from build123d import *

# Parameters (mm, degrees)
F0_W           = 80
F0_H           = 80
F1_DEPTH       = 80
F3_DEPTH       = 86.9
F4_W           = 8
F4_H           = 80
F5_DEPTH       = 25
F6_W           = 30
F6_H           = 25
F7_DEPTH       = 25
F9_DEPTH       = 50.3
F11_W          = 223.7579002976
F11_H          = 231.868326664
F12_DEPTH      = 25
F13_W          = 207.2095647454
F13_H          = 262.1310725808
F14_DEPTH      = 25
F16_DEPTH      = 127.5
F18_DEPTH      = 40.001
F18_DEPTH_BACK = 40.001


# Not quite as in the source:
# - a feature of the source that left no trace in its solid (it failed there, or was rolled back) is left out


with BuildPart() as f1:
    # F0 (on Top) → F1 (new body)
    with BuildSketch(Plane.XY):
        Rectangle(F0_W, F0_H)
    extrude(amount=F1_DEPTH)

    # F2 (on face) → F3 (cut)
    with BuildSketch(Plane.XZ.offset(40)):
        Polygon((-40, 28.6014117301), (0, 80), (-40, 80), align=None)
    extrude(amount=-F3_DEPTH, mode=Mode.SUBTRACT)

    # F4 (on face) → F5 (cut)
    with BuildSketch(Plane.XY.offset(80)):
        with Locations((9.4103766605, 0)):
            Rectangle(F4_W, F4_H)
    extrude(amount=-F5_DEPTH, mode=Mode.SUBTRACT)

    # F6 (on face) → F7 (cut)
    with BuildSketch(Plane.YZ.offset(5.4103766605)):
        with Locations((-25, 67.5)):
            Rectangle(F6_W, F6_H)
        with Locations((25, 67.5)):
            Rectangle(F6_W, F6_H)
    extrude(amount=-F7_DEPTH, mode=Mode.SUBTRACT)

    # F8 (on face) → F9 (cut)
    with BuildSketch(Plane(origin=(-40, 0, 0), x_dir=(0, -1, 0), z_dir=(-1, 0, 0))):
        Polygon((-10.1708276197, 55.0271123648), (0, 80.8042436838), (10.1708276197, 55.0271123648), (61.0520653427, 55.0271123648), (61.0520653427, 88.9606252313), (0, 88.9606252313), (-61.0520653427, 88.9606252313), (-61.0520653427, 55.0271123648), align=None)
    extrude(amount=-F9_DEPTH, mode=Mode.SUBTRACT)

    # F11 (on face) → F12 (cut)
    with BuildSketch(Plane(origin=(-23.8023577799, -28.0559598365, 29.5937245096), x_dir=(0.8636441264, -0.3468224195, 0.3658319728), z_dir=(-0.5041019966, -0.5941875801, 0.6267553723))):
        with Locations((27.8940685093, 6.7206919193)):
            Rectangle(F11_W, F11_H)
    extrude(amount=F12_DEPTH, mode=Mode.SUBTRACT)

    # F13 (on face) → F14 (cut)
    with BuildSketch(Plane(origin=(-23.8023577799, 28.0559598365, 29.5937245096), x_dir=(0.8636441264, 0.3468224195, 0.3658319728), z_dir=(-0.5041019966, 0.5941875801, 0.6267553723))):
        with Locations((8.8918171823, -6.4797215164)):
            Rectangle(F13_W, F13_H)
    extrude(amount=F14_DEPTH, mode=Mode.SUBTRACT)

    # F15 (on face) → F16 (cut)
    with BuildSketch(Plane.XZ.offset(40)):
        Polygon((30, 0), (30, 48.7106099482), (-30.5624192708, 0), align=None)
    extrude(amount=-F16_DEPTH, mode=Mode.SUBTRACT)

    # F17 (on Right) → F18 (cut, two sides)
    with BuildSketch(Plane.YZ) as f18_sk:
        Polygon((15.2906342708, 28.7791552365), (0, 67.5320180601), (-15.3222406511, 28.6990514489), (-15.3607661463, 28.6014117301), (15.3607661463, 28.6014117301), align=None)
        Polygon((26.6459640524, 0), (15.3607661463, 28.6014117301), (-15.3607661463, 28.6014117301), (-26.6459640524, 0), align=None)
    extrude(amount=-F18_DEPTH, mode=Mode.SUBTRACT)
    extrude(f18_sk.sketch, amount=F18_DEPTH_BACK, mode=Mode.SUBTRACT)


solid = f1.part
For this review, take the finished solid that the model builds, in its own axes (mm). A direction names the side the tool comes from. Round coordinates to 2 decimals unless told otherwise and drop trailing zeros. Order: outer loops, then holes, each group sorted by start corner. A loop starts at its lowest first (then second) coordinate and runs counter-clockwise, first axis right, second up. Notation, with made-up numbers: (0.5, 59) -> (44.5, 59) arc R23 ccw to (44.5, 96) -> close; hole circle Ø4 at (82.5, 43.25). An arc over 180 degrees is marked (long way). Write item = value, one per line. Start each with the question number.
1) Tool access review of faces 4 (the face through (0.189, -7.353, 62.17)), 5 (the face through (13.41, 0, 68)), 6 (the face through (30, -28, 29)), 7 (the face through (0.2, 7.5, 61.8)): name each direction out of +Z, -Z, +X, -X, +Y, -Y from which nothing blocks a thin tool from reaching the whole face with its end or side.
2) Take a section at C-C on y = 12.5. State the section outline as (x, z) points, plus the area to 3 significant figures.
3) The part is to be moulded in two halves that separate along X. For faces 1 (the face through (6.872, -27.56, 30.109)), 2 (the face through (-40, 29, 10)), 3 (the face through (-35, 33, 0)), say which applies: +X half, -X half, draft (parallel to the pull), parting line (faces both ways), or undercut.
4) Take a section at D-D on x = -7.5. State the section outline as (y, z) points, plus the area to 3 significant figures.
5) Insertion check: pin 1 (6 mm diameter, centred on x = 26, y = 21.5, fed in from -Z); pin 2 (3 mm diameter, centred on y = 30.5, z = 24.5, fed in from -X); pin 3 (10 mm diameter, centred on x = -28.5, z = 35.5, fed in from -Y). Each pin has a flat end and moves straight along its axis. Give the tip position at first contact, or say it passes through.
6) Take a section at A-A on x = -19.5. State the section outline as (y, z) points.
7) Take a section at B-B on z = 45.5. State the section outline as (x, y) points, plus the area to 3 significant figures.
8) To check wall thickness, follow line 1 (X direction, y = 8.5, z = 69.5); line 2 (X direction, y = -34.5, z = 30); line 3 (X direction, y = 5.5, z = 66). State the ranges of each line that lie inside material, in increasing order. Write a range as from..to.
Verdict:
q1.face_4 = +Z, -X, -Y
q1.face_5 = +Z, +Y, -Y
q1.face_6 = -Z, +Y, -Y
q1.face_7 = +Z, -X, +Y
q2.outline = (-34.36, 35.85) -> (14.01, 35.85) -> (30, 48.71) -> (30, 35.85) -> (40, 35.85) -> (40, 80) -> (20.53, 80) -> (13.41, 74.27) -> (13.41, 55) -> (-10.55, 55) -> close
q2.area = 1,740 mm2
q3.face_1 = undercut
q3.face_2 = -X half
q3.face_3 = draft
q4.outline = (-40, 18.55) -> (-19.33, 18.55) -> (0, 67.53) -> (19.33, 18.55) -> (40, 18.55) -> (40, 31.38) -> (15.09, 55) -> (10, 55) -> (10, 55.46) -> (7.25, 62.43) -> (0, 69.3) -> (-7.25, 62.43) -> (-10, 55.46) -> (-10, 55) -> (-15.09, 55) -> (-40, 31.38) -> close
q4.area = 1,560 mm2
q5.pin_1 = 43.08
q5.pin_2 = -29.82
q5.pin_3 = -24.61
q6.outline = (-40, 8.9) -> (-23.14, 8.9) -> (-4.97, 54.94) -> (-40, 21.73) -> close; (4.97, 54.94) -> (23.14, 8.9) -> (40, 8.9) -> (40, 21.73) -> close
q7.outline = (-26.85, -8.69) -> (10.05, -40) -> (26.01, -40) -> (26.01, -8.69) -> close; (-26.85, 8.69) -> (26.01, 8.69) -> (26.01, 40) -> (10.05, 40) -> close; (30, -40) -> (40, -40) -> (40, -8.69) -> (30, -8.69) -> close; (30, 8.69) -> (40, 8.69) -> (40, 40) -> (30, 40) -> close
q7.area = 2,780 mm2
q8.line_1 = 13.41..40
q8.line_2 = -15.7..6.74, 30..40
q8.line_3 = -5.12..5.41, 13.41..40
